Work out the finished part from the listing and answer in its coordinate system (mm). A direction names the side the tool comes from. Give positions to 0.01 mm unless a question says otherwise; leave off trailing zeros. Loops run counter-clockwise (first coordinate to the right, second up) from the corner with the lowest first, then second, coordinate; pieces in that order, holes last. Notation, with made-up numbers: M -10,80 L 28,80 A21 ccw 28,91 Z; hole C 26.25,-18.5 d1. An arc over 180 degrees is marked long. Answer in a Markdown table with one row per item. Add a question column.
from build123d import *

# Parameters (mm, degrees)
SKETCH1_R                                       = 8
BOSS_EXTRUDE1_DEPTH                             = 18
SKETCH3_R                                       = 8
BOSS_EXTRUDE2_DEPTH                             = 23
BOSS_EXTRUDE3_DEPTH                             = 8
CSK_FOR_M5_FLAT_HEAD_MACHINE_SCREW1_D           = 5.5
CSK_FOR_M5_FLAT_HEAD_MACHINE_SCREW1_CSINK_D     = 11.2
CSK_FOR_M5_FLAT_HEAD_MACHINE_SCREW1_CSINK_ANGLE = 90


with BuildPart() as part:
    # Sketch1 → Boss-Extrude1 (new body)
    with BuildSketch(Plane.YZ):
        Circle(SKETCH1_R)
    extrude(amount=BOSS_EXTRUDE1_DEPTH)



with BuildPart() as body_2:
    # Sketch3 → Boss-Extrude2 (new body)
    with BuildSketch(Plane(origin=(81, 0, 0), x_dir=(0, 0, -1), z_dir=(1, 0, 0))):
        Circle(SKETCH3_R)
    extrude(amount=BOSS_EXTRUDE2_DEPTH)


with BuildPart() as part_1:
    add(part.part)

    add(body_2.part)  # Boss-Extrude3 merges body 2
    # Sketch7 → Boss-Extrude3 (add, symmetric)
    with BuildSketch(Plane(origin=(0, 0, 0), x_dir=(-1, 0, 0), z_dir=(0, 1, 0))):
        with BuildLine():
            Line((0, 0), (0, -13))
            ThreePointArc((0, -13), (-5.272077939, -25.727922061), (-18, -31))
            Line((-18, -31), (-77, -31))
            ThreePointArc((-77, -31), (-89.727922061, -25.727922061), (-95, -13))
            Line((-95, -13), (-95, 0))
            Line((-95, 0), (-81, 0))
            Line((-81, 0), (-81, -8))
            ThreePointArc((-81, -8), (-78.949747468, -12.949747468), (-74, -15))
            Line((-74, -15), (-25, -15))
            ThreePointArc((-25, -15), (-20.050252532, -12.949747468), (-18, -8))
            Line((-18, -8), (-18, 0))
            Line((-18, 0), (0, 0))
        make_face()
    extrude(amount=BOSS_EXTRUDE3_DEPTH, both=True)

    # CSK for M5 Flat Head Machine Screw1 (through all)
    with Locations(Plane.YZ.offset(104)):
        with Locations((0, 0)):
            CounterSinkHole(CSK_FOR_M5_FLAT_HEAD_MACHINE_SCREW1_D / 2, CSK_FOR_M5_FLAT_HEAD_MACHINE_SCREW1_CSINK_D / 2, counter_sink_angle=CSK_FOR_M5_FLAT_HEAD_MACHINE_SCREW1_CSINK_ANGLE)


solid = part_1.part
(1) The mould has two halves that part along X. Classify faces 4 (the face through (104, 5.45, 1.89)), 5 (the face through (81, 0, -3)), 6 (the face through (47, -8, -19)): pulls with the +X half, pulls with the -X half, needs draft (parallel to the pull), parting line crosses it, or undercut.
(2) Section B-B, the plane z = -10 is taken. Determine the outline of the cut face in (x, y), and give its area (3 significant figures).
(3) Section C-C, the plane x = 59 is taken. Determine the outline of the cut face in (y, z), and give its area (3 significant figures).
(4) Each of these flat-tipped pins is pushed along its axis until it touches: P1, Ø5, axis at x = 51.5, y = 2.5, coming from the +Z side; P2, Ø1, axis at y = -4, z = -22, coming from the -X side; P3, Ø3.5, axis at y = 0, z = 0, coming from the -X side; P4, Ø6, axis at x = 89, y = 4, coming from the +Z side. Where does it stop, or does it pass through?
(5) Section A-A, the plane y = 0 is taken. Determine the outline of the cut face in (x, z).
(6) Which of the six approach directions +Z, -Z, +X, -X, +Y, -Y give full straight-line access (tool end or side, diameter ignored) to faces 1 (the face through (95, 0, 8)), 2 (the face through (50, 0, -15)), 3 (the face through (47, 8, -19))?
(7) Consider line 1 along X through (y, z) = (7.25, -7); line 2 along X through (y, z) = (-6.75, 0.5); line 3 along Y through (x, z) = (87.5, 0). Determine where each line is inside the solid, lowest interval first. Write a range as from..to.
(8) Section D-D, the plane x = 91 is taken. Determine the outline of the cut face in (y, z), and give its area (3 significant figures).
Numbers:
| question | item | result |
|---|---|---|
| 1 | face 4 | pulls with the +X half |
| 1 | face 5 | undercut |
| 1 | face 6 | needs draft |
| 2 | outline | M 0,-8 L 18.29,-8 L 18.29,8 L 0,8 Z; M 80.71,-8 L 95,-8 L 95,8 L 80.71,8 Z |
| 2 | area | 521 mm² |
| 3 | outline | M -8,-31 L 8,-31 L 8,-15 L -8,-15 Z |
| 3 | area | 256 mm² |
| 4 | P1 | stops at z = -15 |
| 4 | P2 | stops at x = 2.13 |
| 4 | P3 | passes through |
| 4 | P4 | stops at z = 7.94 |
| 5 | outline | M 0,-13 A18 ccw 18,-31 L 77,-31 A18 ccw 95,-13 L 95,-8 L 104,-8 L 104,-5.6 L 101.15,-2.75 L 81,-2.75 L 81,-8 A7 cw 74,-15 L 25,-15 A7 cw 18,-8 L 18,-2.75 L 0,-2.75 Z; M 0,2.75 L 18,2.75 L 18,8 L 0,8 Z; M 81,2.75 L 101.15,2.75 L 104,5.6 L 104,8 L 81,8 Z |
| 6 | face 1 | +X |
| 6 | face 2 | +Z, +Y, -Y |
| 6 | face 3 | +Z, -Z, +X, -X, +Y |
| 7 | line 1 | x = 0..18, 81..95 |
| 7 | line 2 | x = 0..18, 81..104 |
| 7 | line 3 | y = -8..-2.75, 2.75..8 |
| 8 | outline | M -8,-24.31 L 8,-24.31 L 8,0 A8 ccw -8,0 Z; hole C 0,0 d5.5 |
| 8 | area | 466 mm² |
